from build123d import *

# Parameters (mm, degrees)
F0_W     = 20
F0_H     = 3
F1_DEPTH = 30
F2_W     = 3
F2_H     = 10
F3_DEPTH = 3
F4_W     = 3
F4_H     = 10
F5_DEPTH = 3


with BuildPart() as f1:
    # F0 (on Top) → F1 (new body)
    with BuildSketch(Plane.XY):
        with Locations((10.308956, 0.197368)):
            Rectangle(F0_W, F0_H)
    extrude(amount=F1_DEPTH)

    # F2 (on face) → F3 (join)
    with BuildSketch(Plane.YZ.offset(20.308956)):
        with Locations((0.197368, 25)):
            Rectangle(F2_W, F2_H)
        with Locations((0.197368, 5)):
            Rectangle(F2_W, F2_H)
    extrude(amount=F3_DEPTH)

    # F4 (on face) → F5 (join)
    with BuildSketch(Plane(origin=(0.308956, 0, 0), x_dir=(0, -1, 0), z_dir=(-1, 0, 0))):
        with Locations((-0.197368, 15)):
            Rectangle(F4_W, F4_H)
    extrude(amount=F5_DEPTH)


solid = f1.part
Read the model definition and answer for the solid it produces. Units are mm, in the model's axes. A direction names the side the tool comes from. Coordinates: 2 decimals unless noted, no trailing zeros. Order: outer loops, then holes, each group sorted by start corner. A loop starts at its lowest first (then second) coordinate and runs counter-clockwise, first axis right, second up. Notation, with made-up numbers: (17.5, 75) -> (31.5, 75) arc R8 ccw to (31.5, 88) -> close; hole circle Ø2 at (55.5, 71.5). An arc over 180 degrees is marked (long way). Answer as a JSON object with one key per item and string values.
1) The mould has two halves that part along Z. Classify faces 6 (the face through (22, 0, 20)), 7 (the face through (12, 0, 30)), 8 (the face through (-2.691, 0, 15)): released by +Z, released by -Z, zero draft, split by the parting line, or undercut.
Model answer:
{"face 6": "undercut", "face 7": "released by +Z", "face 8": "zero draft"}
2) A cutting plane is placed at C-C, the plane z = 22. Determine the outline of the cut face in (x, y).
Model answer:
{"outline": "(0.31, -1.3) -> (23.31, -1.3) -> (23.31, 1.7) -> (0.31, 1.7) -> close"}
3) Consider line 1 along Z through (x, y) = (22.25, 1.05); line 2 along X through (y, z) = (0.95, 10.25); line 3 along X through (y, z) = (-0.95, 9). Determine where each line is inside the solid, lowest interval first. Write a range as from..to.
Model answer:
{"line 1": "z = 0..10, 20..30", "line 2": "x = -2.69..20.31", "line 3": "x = 0.31..23.31"}
4) A cutting plane is placed at A-A, the plane y = 0.6. Determine the outline of the cut face in (x, z).
Model answer:
{"outline": "(-2.69, 10) -> (0.31, 10) -> (0.31, 0) -> (23.31, 0) -> (23.31, 10) -> (20.31, 10) -> (20.31, 20) -> (23.31, 20) -> (23.31, 30) -> (0.31, 30) -> (0.31, 20) -> (-2.69, 20) -> close"}
5) A tool of negligible diameter and unlimited length cuts with its end or side. For faces 1 (the face through (0.309, 0, 5)), 2 (the face through (-1, 0, 20)), 3 (the face through (23.309, 0, 25)), 4 (the face through (20.309, 0, 15)), 5 (the face through (10, 1.697, 15)), from which of +Z, -Z, +X, -X, +Y, -Y can it reach the whole face along a straight path? Write none if from no direction.
Model answer:
{"face 1": "-Z, -X, +Y, -Y", "face 2": "+Z, -X, +Y, -Y", "face 3": "+Z, -Z, +X, +Y, -Y", "face 4": "+X, +Y, -Y", "face 5": "+Z, -Z, +X, -X, +Y"}
6) Each of these flat-tipped pins is pushed along its axis until it touches: pin 1 (0.9 mm diameter, centred on x = -1, y = -0.5, fed in from -Z); pin 2 (1 mm diameter, centred on y = 1, z = 9, fed in from -X). Where does it stop, or does it pass through?
Model answer:
{"pin 1": "stops at z = 10", "pin 2": "stops at x = 0.31"}
7) A cutting plane is placed at B-B, the plane x = -0.5. Determine the outline of the cut face in (y, z).
Model answer:
{"outline": "(-1.3, 10) -> (1.7, 10) -> (1.7, 20) -> (-1.3, 20) -> close"}
